For this review, take the finished solid that the model builds, in its own axes (mm). A direction names the side the tool comes from. Give positions to 0.01 mm unless a question says otherwise; leave off trailing zeros. Write each loop counter-clockwise with the first axis right and the second up, starting at its lowest first coordinate (ties: lowest second). Pieces come first, ordered by that corner, then holes. Notation, with made-up numbers: M -22,28 L -18,28 A12 cw -18,32 Z; hole C 26.5,18 d3. An arc over 180 degrees is marked long. Write item = value, one per line.
```python
from build123d import *

# Parameters (mm, degrees)
F1_DEPTH = 3.302
F2_DEPTH = 1.905
F3_DEPTH = 39.751


with BuildPart() as f1:
    # F0 (on Top) → F1 (new body)
    with BuildSketch(Plane.XY):
        with BuildLine():
            Line((3.0691199537, 0.762), (4.4822904368, 0.762))
            ThreePointArc((4.4822904368, 0.762), (0, 4.5466), (-4.4822904368, 0.762))
            Line((-4.4822904368, 0.762), (-3.0691199537, 0.762))
            ThreePointArc((-3.0691199537, 0.762), (0, 3.1623), (3.0691199537, 0.762))
        make_face()
        with BuildLine():
            Line((-3.0691199537, 0.762), (3.0691199537, 0.762))
            ThreePointArc((3.0691199537, 0.762), (0, 3.1623), (-3.0691199537, 0.762))
        make_face()
    extrude(amount=F1_DEPTH)



with BuildPart() as f1b:
    # F0 (on Top) → F1, piece 2 (new body)
    with BuildSketch(Plane.XY):
        with BuildLine():
            Line((3.0691199537, -0.762), (-3.0691199537, -0.762))
            ThreePointArc((-3.0691199537, -0.762), (0, -3.1623), (3.0691199537, -0.762))
        make_face()
        with BuildLine():
            ThreePointArc((-4.4822904368, -0.762), (0, -4.5466), (4.4822904368, -0.762))
            Line((4.4822904368, -0.762), (3.0691199537, -0.762))
            ThreePointArc((3.0691199537, -0.762), (0, -3.1623), (-3.0691199537, -0.762))
            Line((-3.0691199537, -0.762), (-4.4822904368, -0.762))
        make_face()
    extrude(amount=F1_DEPTH)


with BuildPart() as f1_1:
    add(f1.part)

    add(f1b.part)  # F2 merges F1b
    # F0 (on Top) → F2 (join)
    with BuildSketch(Plane.XY):
        with BuildLine():
            ThreePointArc((3.1623, 0), (3.1389185494, 0.3838380261), (3.0691199537, 0.762))
            Line((3.0691199537, 0.762), (-3.0691199537, 0.762))
            ThreePointArc((-3.0691199537, 0.762), (-3.1623, 0), (-3.0691199537, -0.762))
            Line((-3.0691199537, -0.762), (3.0691199537, -0.762))
            ThreePointArc((3.0691199537, -0.762), (3.1389185494, -0.3838380261), (3.1623, 0))
        make_face()
        with BuildLine():
            ThreePointArc((4.5466, 0), (4.5304940823, 0.3823544559), (4.4822904368, 0.762))
            Line((4.4822904368, 0.762), (3.0691199537, 0.762))
            ThreePointArc((3.0691199537, 0.762), (3.1389185494, 0.3838380261), (3.1623, 0))
            ThreePointArc((3.1623, 0), (3.1389185494, -0.3838380261), (3.0691199537, -0.762))
            Line((3.0691199537, -0.762), (4.4822904368, -0.762))
            ThreePointArc((4.4822904368, -0.762), (4.5304940823, -0.3823544559), (4.5466, 0))
        make_face()
        with BuildLine():
            Line((-3.0691199537, 0.762), (-4.4822904368, 0.762))
            ThreePointArc((-4.4822904368, 0.762), (-4.5466, 0), (-4.4822904368, -0.762))
            Line((-4.4822904368, -0.762), (-3.0691199537, -0.762))
            ThreePointArc((-3.0691199537, -0.762), (-3.1623, 0), (-3.0691199537, 0.762))
        make_face()
    extrude(amount=F2_DEPTH)

    # F0 (on Top) → F3 (join)
    with BuildSketch(Plane.XY):
        with BuildLine():
            Line((-3.0691199537, 0.762), (3.0691199537, 0.762))
            ThreePointArc((3.0691199537, 0.762), (0, 3.1623), (-3.0691199537, 0.762))
        make_face()
        with BuildLine():
            ThreePointArc((3.1623, 0), (3.1389185494, 0.3838380261), (3.0691199537, 0.762))
            Line((3.0691199537, 0.762), (-3.0691199537, 0.762))
            ThreePointArc((-3.0691199537, 0.762), (-3.1623, 0), (-3.0691199537, -0.762))
            Line((-3.0691199537, -0.762), (3.0691199537, -0.762))
            ThreePointArc((3.0691199537, -0.762), (3.1389185494, -0.3838380261), (3.1623, 0))
        make_face()
        with BuildLine():
            Line((3.0691199537, -0.762), (-3.0691199537, -0.762))
            ThreePointArc((-3.0691199537, -0.762), (0, -3.1623), (3.0691199537, -0.762))
        make_face()
    extrude(amount=-F3_DEPTH)


solid = f1_1.part
```
1. Insertion check: P1, Ø3, axis at x = 1.5, z = -12.5, coming from the -Y side; P2, Ø2, axis at x = 1.5, z = -17, coming from the +Y side; P3, Ø1, axis at y = 0, z = -12.5, coming from the +X side. Each pin has a flat end and moves straight along its axis. Give the tip position at first contact, or say it passes through.
Responses:
P1 = -3.16
P2 = 3.12
P3 = 3.16
2. The part is to be moulded in two halves that separate along Y. For faces 1 (the face through (0, -2, 3.302)), 2 (the face through (0, -0.762, 3)), 3 (the face through (0, 0, 1.905)), say which applies: +Y half, -Y half, draft (parallel to the pull), parting line (faces both ways), or undercut.
Responses:
face_1 = draft
face_2 = undercut
face_3 = undercut
3. For line 1 along Z through (x, y) = (-2.75, -2.25); line 2 along Y through (x, z) = (2, -15); line 3 along Y through (x, z) = (1.75, 0.5), list the stretches that pass through material, from the lowest coordinate up. Write a range as from..to.
Responses:
line_1 = 0..3.3
line_2 = -2.45..2.45
line_3 = -4.2..4.2
4. We need section A-A, the plane z = -28. Write out the cut boundary in (x, y), then the cut area to 3 significant figures.
Responses:
outline = C 0,0 d6.32
area = 31.4 mm2
5. We need section D-D, the plane x = 0.75. Write out the cut boundary in (y, z) (3 decimals), then the cut area to 3 significant figures.
Responses:
outline = M -4.484,0 L -3.072,0 L -3.072,-39.751 L 3.072,-39.751 L 3.072,0 L 4.484,0 L 4.484,3.302 L 0.762,3.302 L 0.762,1.905 L -0.762,1.905 L -0.762,3.302 L -4.484,3.302 Z
area = 272 mm2
6. Machinability: for faces 4 (the face through (0, 0.762, 3)), 5 (the face through (2, -3, 0)), 6 (the face through (0, 2, 3.302)), which of the approach directions +Z, -Z, +X, -X, +Y, -Y give a long, thin tool a straight path to every point of the face, cutting with its end or side? Answer none if there is none.
Responses:
face_4 = +Z, +X, -X
face_5 = -Z
face_6 = +Z, +X, -X, +Y, -Y
7. We need section B-B, the plane y = 1.5. Write out the cut boundary in (x, z).
Responses:
outline = M -4.29,0 L -2.78,0 L -2.78,-39.75 L 2.78,-39.75 L 2.78,0 L 4.29,0 L 4.29,3.3 L -4.29,3.3 Z
8. We need section C-C, the plane x = 2.5. Write out the cut boundary in (y, z) (3 decimals).
Responses:
outline = M -3.798,0 L -1.937,0 L -1.937,-39.751 L 1.937,-39.751 L 1.937,0 L 3.798,0 L 3.798,3.302 L 0.762,3.302 L 0.762,1.905 L -0.762,1.905 L -0.762,3.302 L -3.798,3.302 Z
